```python
from build123d import *

# Parameters (mm, degrees)
F0_W      = 56
F0_H      = 45
F1_DEPTH  = 2
F2_W      = 56
F2_H      = 20
F3_DEPTH  = 2
F4_W      = 56
F4_H      = 2
F5_DEPTH  = 20
F6_W      = 56
F6_H      = 2
F7_DEPTH  = 20
F9_W      = 69.615941
F9_H      = 33.992227
F10_DEPTH = 25


with BuildPart() as f1:
    # F0 (on Top) → F1 (new body)
    with BuildSketch(Plane.XY):
        Rectangle(F0_W, F0_H)
    extrude(amount=F1_DEPTH)

    # F2 (on face) → F3 (join)
    with BuildSketch(Plane(origin=(0, 0, 0), x_dir=(1, 0, 0), z_dir=(0, 0, -1))):
        with Locations((0, -12.5)):
            Rectangle(F2_W, F2_H)
    extrude(amount=F3_DEPTH)

    # F4 (on face) → F5 (join)
    with BuildSketch(Plane(origin=(0, 0, -2), x_dir=(1, 0, 0), z_dir=(0, 0, -1))):
        with Locations((0, -3.5)):
            Rectangle(F4_W, F4_H)
    extrude(amount=F5_DEPTH)

    # F6 (on face) → F7 (join)
    with BuildSketch(Plane(origin=(0, 4.5, 0), x_dir=(-1, 0, 0), z_dir=(0, 1, 0))):
        with Locations((0, -21)):
            Rectangle(F6_W, F6_H)
    extrude(amount=F7_DEPTH)

    # F9 (on offset) → F10 (cut)
    with BuildSketch(Plane(origin=(0, 22.5, 0), x_dir=(-1, 0, 0), z_dir=(0, 1, 0))):
        with Locations((-4.858752, -12.837998)):
            Rectangle(F9_W, F9_H)
    extrude(amount=F10_DEPTH, mode=Mode.SUBTRACT)


solid = f1.part
```
Can you work these out from the model? Positions are in its coordinate system, mm. A direction names the side the tool comes from. Coordinates: 2 decimals unless noted, no trailing zeros. Loops run counter-clockwise (first coordinate to the right, second up) from the corner with the lowest first, then second, coordinate; pieces in that order, holes last.
1) Imagine slicing it at B-B on z = -6.25. List the corners of the cut face in (x, y) for me.
2) Thinking about a two-plate mould opening in Z: for faces 4 (the flat face through (0, 13, -2)), 5 (the flat face through (0, 2.5, -11)), 6 (the flat face through (0, 0, 2)), which applies, pulls with the +Z half, pulls with the -Z half, needs draft (parallel to the pull), parting line crosses it, or undercut?
3) I need wall thicknesses on probe 1 along Z at (x, y) = (-2, 5); probe 2 along Z at (x, y) = (18.5, -19); probe 3 along Y at (x, z) = (-4.5, -8.5). Which ranges of each line are inside material? Lowest first, please.
4) Imagine slicing it at C-C on y = -17.5. List the corners of the cut face in (x, z) for me.
5) Imagine slicing it at A-A on x = -22. List the corners of the cut face in (y, z) for me, plus the area to 3 significant figures.
6) Which directions (+Z, -Z, +X, -X, +Y, -Y) give clear straight access to the entire face, cutting with the end or side of a thin tool? Please do faces 1 (the flat face through (0, 13, -20)), 2 (the flat face through (0, -10, 0)), 3 (the flat face through (0, 12, -22)).
7) For pin 1 (3 mm diameter, centred on x = -19, z = -13.5, fed in from +Y); pin 2 (7.5 mm diameter, centred on x = 2, y = -14.5, fed in from -Z); pin 3 (5 mm diameter, centred on x = -6.5, z = -2, fed in from -Y), each with a flat end and sliding along its axis, tell me the tip position at first contact or that it passes through.
Completed:
1. outline: (-28, 2.5) - (28, 2.5) - (28, 4.5) - (-28, 4.5) - close
2. face 4: undercut
2. face 5: needs draft
2. face 6: pulls with the +Z half
3. probe 1: z = -22 to -20, -2 to 2
3. probe 2: z = 0 to 2
3. probe 3: y = 2.5 to 4.5
4. outline: (-28, 0) - (28, 0) - (28, 2) - (-28, 2) - close
5. outline: (-22.5, 0) - (2.5, 0) - (2.5, -22) - (22.5, -22) - (22.5, -20) - (4.5, -20) - (4.5, -2) - (22.5, -2) - (22.5, 2) - (-22.5, 2) - close
5. area: 206 mm2
6. face 1: +X, -X, +Y
6. face 2: -Z, +X, -X, -Y
6. face 3: -Z, +X, -X, +Y, -Y
7. pin 1: stops at y = 4.5
7. pin 2: stops at z = 0
7. pin 3: stops at y = -22.5
